from build123d import *

# Parameters (mm, degrees)
PAD005_DEPTH        = 15
HOLE001_D           = 3
HOLE001_DEPTH       = 25
HOLE001_CSINK_D     = 6.1
HOLE001_CSINK_ANGLE = 90
HOLE_D              = 3
HOLE_DEPTH          = 25
HOLE_CSINK_D        = 6.1
HOLE_CSINK_ANGLE    = 90


with BuildPart() as part:
    # Sketch005 (on Face53 of Binder002) → Pad005 (new body)
    with BuildSketch(Plane(origin=(87.2, 0, 0), x_dir=(0, -1, 0), z_dir=(-1, 0, 0))):
        Polygon((-57.53, -4.827157), (-57.53, -1.01), (-45.53, -1.01), (-45.53, -12.584517), (-44.204517, -13.91), (0, -13.91), (0, -16.91), (-45.447157, -16.91), align=None)
    pad005 = extrude(amount=PAD005_DEPTH)

    # Mirrored: Pad005 across Sketch005 V_Axis
    add(pad005.mirror(Plane(origin=(87.2, 0, 0), x_dir=(-1, 0, 0), z_dir=(0, -1, 0))))

    # Hole001
    with Locations(Plane.XY.offset(-13.91)):
        with Locations((79.7, 39.204517), (79.7, -39.204517)):
            CounterSinkHole(HOLE001_D / 2, HOLE001_CSINK_D / 2, depth=HOLE001_DEPTH, counter_sink_angle=HOLE001_CSINK_ANGLE)

    # Hole
    with Locations(Plane.XY.offset(-13.91)):
        with Locations((79.7, 39.204517), (79.7, -39.204517)):
            CounterSinkHole(HOLE_D / 2, HOLE_CSINK_D / 2, depth=HOLE_DEPTH, counter_sink_angle=HOLE_CSINK_ANGLE)


with BuildPart() as part_1:
    # Body003 placement: moved
    add(part.part.moved(Location((-125, 0, 0))))


solid = part_1.part
Verification items for the finished model (mm, model axes). A direction names the side the tool comes from. Give positions to 0.01 mm unless a question says otherwise; leave off trailing zeros. Order: outer loops, then holes, each group sorted by start corner. A loop starts at its lowest first (then second) coordinate and runs counter-clockwise, first axis right, second up. Notation, with made-up numbers: M 86.5,19.5 L 97.5,19.5 A14 ccw 97.5,36.5 Z; hole C 28.25,28 d6. An arc over 180 degrees is marked long. Answer as a JSON object with one key per item and string values. Group by question number.
1) Mould release check, pull along Y, two halves, no side actions. Record for faces 1 (the face through (-46.73, 39.66, -16.2)), 2 (the face through (-45, 57.53, -3)), 3 (the face through (-45.195, -51.404, -10.953)): released by +Y, released by -Y, zero draft, split by the parting line, or undercut.
2) Scan lines: line 1 along Y through (x, z) = (-45, -4.5); line 2 along Y through (x, z) = (-45.3, -16.05); line 3 along Y through (x, z) = (-45.3, -15.8). Record each from-to range of solid material in increasing order. Write a range as [from, to].
3) Cross-section at A-A (x = -45.3). Enter the section's corners in (y, z), then the cut area to 3 significant figures.
4) Cross-section at B-B (z = -2.5). Enter the section's corners in (x, y).
5) Access from +Z, -Z, +X, -X, +Y, -Y to the whole of each face (thin tool, end or side, straight path). Record for faces 4 (the face through (-46.686, -39.779, -16.195)), 5 (the face through (-45, 45.53, -7)).
6) Depth check by flat-ended pin: pin 1 Ø2 at (x, z) = (-48, -13.5) entering from -Y; pin 2 Ø5 at (x, z) = (-46.5, -12.5) entering from -Y; pin 3 Ø1.5 at (x, y) = (-50.5, -5.5) entering from +Z. Enter the tip coordinate at first touch or a pass-through.
7) Cross-section at D-D (z = -10.75). Enter the section's corners in (x, y).
8) Cross-section at C-C (x = -50). Enter the section's corners in (y, z).
Result sheet:
{
 "1": {"face 1": "undercut", "face 2": "released by +Y", "face 3": "released by -Y"},
 "2": {"line 1": "y = [-57.53, -45.53], [45.53, 57.53]", "line 2": "y = [-46.31, -40.7], [-37.7, 37.7], [40.7, 46.31]", "line 3": "y = [-46.56, -40.7], [-37.7, 37.7], [40.7, 46.56]"},
 "3": {"outline": "M -57.53,-4.83 L -45.45,-16.91 L -40.7,-16.91 L -40.7,-15.46 L -42.25,-13.91 L -44.2,-13.91 L -45.53,-12.58 L -45.53,-1.01 L -57.53,-1.01 Z; M -37.7,-16.91 L 37.7,-16.91 L 37.7,-15.46 L 36.15,-13.91 L -36.15,-13.91 L -37.7,-15.46 Z; M 40.7,-16.91 L 45.45,-16.91 L 57.53,-4.83 L 57.53,-1.01 L 45.53,-1.01 L 45.53,-12.58 L 44.2,-13.91 L 42.25,-13.91 L 40.7,-15.46 Z", "area": "488 mm2"},
 "4": {"outline": "M -52.8,-57.53 L -37.8,-57.53 L -37.8,-45.53 L -52.8,-45.53 Z; M -52.8,45.53 L -37.8,45.53 L -37.8,57.53 L -52.8,57.53 Z"},
 "5": {"face 4": "+Z, -Z", "face 5": "+Z, +X, -X"},
 "6": {"pin 1": "stops at y = -49.86", "pin 2": "stops at y = -52.36", "pin 3": "stops at z = -13.91"},
 "7": {"outline": "M -52.8,-51.61 L -37.8,-51.61 L -37.8,-45.53 L -52.8,-45.53 Z; M -52.8,45.53 L -37.8,45.53 L -37.8,51.61 L -52.8,51.61 Z"},
 "8": {"outline": "M -57.53,-4.83 L -45.45,-16.91 L 45.45,-16.91 L 57.53,-4.83 L 57.53,-1.01 L 45.53,-1.01 L 45.53,-12.58 L 44.2,-13.91 L -44.2,-13.91 L -45.53,-12.58 L -45.53,-1.01 L -57.53,-1.01 Z"}
}
